Could you check a few things on this drawing? It's one solid part, dimensions in mm from its lowest x, y, z. A direction names the side the tool comes from. Coordinates: 2 decimals unless noted, no trailing zeros. Loops run counter-clockwise (first coordinate to the right, second up) from the corner with the lowest first, then second, coordinate; pieces in that order, holes last. Notation, with made-up numbers: (42, -11) -> (75, -11) arc R24 ccw to (75, 0) -> close; hole circle Ø3 at (83.25, -32.5). An arc over 180 degrees is marked (long way). One line per question, with ' | ' between items. Start each with the question number.
(1) Suppose I cut it at C-C (z = 6). Please give me the cut outline in (x, y).
(2) Which directions (+Z, -Z, +X, -X, +Y, -Y) give clear straight access to the entire face, cutting with the end or side of a thin tool? Please do the marked faces 4, 5 and 6.
(3) If we mould it in two halves opening along X, with no side actions, what happens to the marked faces 1, 2 and 3? For each: pulls with the +X half, pulls with the -X half, needs draft (parallel to the pull), parting line crosses it, or undercut.
(4) Suppose I cut it at D-D (x = 47). Please give me the cut outline in (y, z).
(5) I'm going to push flat-ended pins straight in: pin 1 Ø6 at (x, y) = (14, 20.5) entering from +Z; pin 2 Ø2 at (x, z) = (36, 11.5) entering from -Y; pin 3 Ø2 at (y, z) = (10.5, 3) entering from +X; pin 4 Ø4 at (x, y) = (5, 4.5) entering from +Z. Where does each tip first touch, or does it pass through?
(6) Suppose I cut it at B-B (x = 5). Please give me the cut outline in (y, z).
(7) Suppose I cut it at A-A (y = 24.5). Please give me the cut outline in (x, z).
(8) If I drill on line 1 along Y through (x, z) = (5, 2.1); line 2 along Y through (x, z) = (47, 10.5); line 3 along Y through (x, z) = (42, 2.5), over which ranges is the centre line in solid material (lowest first)?
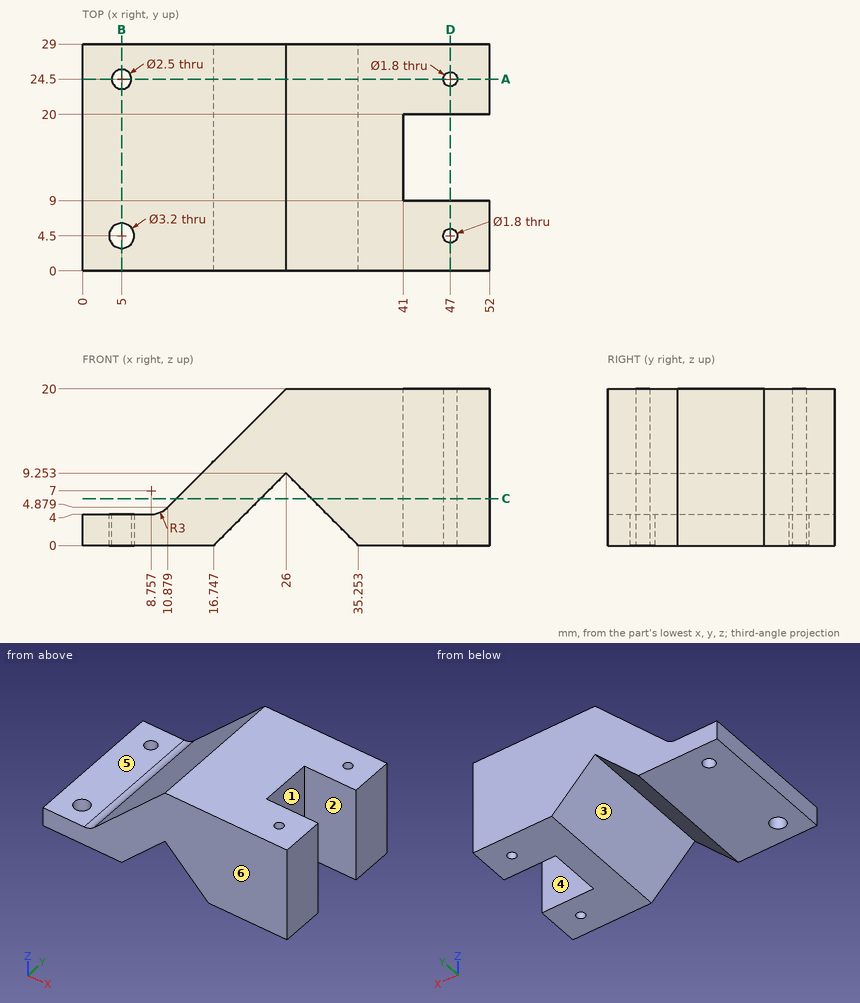
Checks:
1) outline: (12, 0) -> (22.75, 0) -> (22.75, 29) -> (12, 29) -> close; (29.25, 0) -> (52, 0) -> (52, 9) -> (41, 9) -> (41, 20) -> (52, 20) -> (52, 29) -> (29.25, 29) -> close; hole circle Ø1.8 at (47, 4.5); hole circle Ø1.8 at (47, 24.5)
2) face 4: +Z, -Z, +X | face 5: +Z, -X, +Y, -Y | face 6: +Z, -Z, +X, -X, -Y
3) face 1: pulls with the +X half | face 2: needs draft | face 3: undercut
4) outline: (0, 0) -> (3.6, 0) -> (3.6, 20) -> (0, 20) -> close; (5.4, 0) -> (9, 0) -> (9, 20) -> (5.4, 20) -> close; (20, 0) -> (23.6, 0) -> (23.6, 20) -> (20, 20) -> close; (25.4, 0) -> (29, 0) -> (29, 20) -> (25.4, 20) -> close
5) pin 1: stops at z = 11 | pin 2: stops at y = 0 | pin 3: stops at x = 41 | pin 4: stops at z = 4
6) outline: (0, 0) -> (2.9, 0) -> (2.9, 4) -> (0, 4) -> close; (6.1, 0) -> (23.25, 0) -> (23.25, 4) -> (6.1, 4) -> close; (25.75, 0) -> (29, 0) -> (29, 4) -> (25.75, 4) -> close
7) outline: (0, 0) -> (3.75, 0) -> (3.75, 4) -> (0, 4) -> close; (6.25, 0) -> (16.75, 0) -> (26, 9.25) -> (35.25, 0) -> (46.1, 0) -> (46.1, 20) -> (26, 20) -> (10.88, 4.88) arc R3 cw to (8.76, 4) -> (6.25, 4) -> close; (47.9, 0) -> (52, 0) -> (52, 20) -> (47.9, 20) -> close
8) line 1: y = 0 to 2.9, 6.1 to 23.25, 25.75 to 29 | line 2: y = 0 to 3.6, 5.4 to 9, 20 to 23.6, 25.4 to 29 | line 3: y = 0 to 9, 20 to 29
